from build123d import *

# Parameters (mm, degrees)
CYLINDER001_R     = 1.65
CYLINDER001_DEPTH = 10
CYLINDER002_R     = 1.65
CYLINDER002_DEPTH = 10
CYLINDER003_R     = 1.65
CYLINDER003_DEPTH = 10
CYLINDER004_R     = 1.65
CYLINDER004_DEPTH = 10
CYLINDER_R        = 1.65
CYLINDER_DEPTH    = 10
BOX_W             = 50
BOX_H             = 10
BOX_DEPTH         = 3


with BuildPart() as taladro002:
    # Cylinder001 → Cylinder001 (new body)
    with BuildSketch(Plane(origin=(15, 5, -4), x_dir=(1, 0, 0), z_dir=(0, 0, 1))):
        Circle(CYLINDER001_R)
    extrude(amount=CYLINDER001_DEPTH)


with BuildPart() as taladro003:
    # Cylinder002 → Cylinder002 (new body)
    with BuildSketch(Plane(origin=(25, 5, -4), x_dir=(1, 0, 0), z_dir=(0, 0, 1))):
        Circle(CYLINDER002_R)
    extrude(amount=CYLINDER002_DEPTH)


with BuildPart() as taladro004:
    # Cylinder003 → Cylinder003 (new body)
    with BuildSketch(Plane(origin=(35, 5, -4), x_dir=(1, 0, 0), z_dir=(0, 0, 1))):
        Circle(CYLINDER003_R)
    extrude(amount=CYLINDER003_DEPTH)


with BuildPart() as taladro005:
    # Cylinder004 → Cylinder004 (new body)
    with BuildSketch(Plane(origin=(45, 5, -4), x_dir=(1, 0, 0), z_dir=(0, 0, 1))):
        Circle(CYLINDER004_R)
    extrude(amount=CYLINDER004_DEPTH)


with BuildPart() as taladros:
    # Cylinder → Cylinder (new body)
    with BuildSketch(Plane(origin=(5, 5, -4), x_dir=(1, 0, 0), z_dir=(0, 0, 1))):
        Circle(CYLINDER_R)
    extrude(amount=CYLINDER_DEPTH)

    # Fusion: union taladro002, taladro003, taladro004, taladro005
    add(taladro002.part)
    add(taladro003.part)
    add(taladro004.part)
    add(taladro005.part)


with BuildPart() as pieza_final:
    # Box → Box (new body)
    with BuildSketch(Plane.XY):
        with Locations((25, 5)):
            Rectangle(BOX_W, BOX_H)
    extrude(amount=BOX_DEPTH)

    # Cut: cut Taladros
    add(taladros.part, mode=Mode.SUBTRACT)


solid = pieza_final.part
Read the model definition and answer for the solid it produces. Units are mm, in the model's axes. Give positions to 0.01 mm unless a question says otherwise; leave off trailing zeros. Loops run counter-clockwise (first coordinate to the right, second up) from the corner with the lowest first, then second, coordinate; pieces in that order, holes last. Notation, with made-up numbers: M 87.5,-28.75 L 130.5,-28.75 A19 ccw 130.5,6.25 Z; hole C 41.25,-7.5 d11. An arc over 180 degrees is marked long. Write each question's results on one line, items separated by ' | '.
1. Section C-C on x = 35 is taken. Give the vertices of the cut face in (y, z).
Values:
outline: M 0,0 L 3.35,0 L 3.35,3 L 0,3 Z; M 6.65,0 L 10,0 L 10,3 L 6.65,3 Z
2. Straight lines are drawn through the part: line 1 (X direction, y = 5, z = 2.3); line 2 (Y direction, x = 35, z = 1.95); line 3 (X direction, y = 4.25, z = 2.2). For each, find the intervals that lie inside material, in ascending order. Write a range as [from, to].
Values:
line 1: x = [0, 3.35], [6.65, 13.35], [16.65, 23.35], [26.65, 33.35], [36.65, 43.35], [46.65, 50] | line 2: y = [0, 3.35], [6.65, 10] | line 3: x = [0, 3.53], [6.47, 13.53], [16.47, 23.53], [26.47, 33.53], [36.47, 43.53], [46.47, 50]
3. Section A-A on z = 2.4 is taken. Give the vertices of the cut face in (x, y), plus the area to 3 significant figures.
Values:
outline: M 0,0 L 50,0 L 50,10 L 0,10 Z; hole C 5,5 d3.3; hole C 15,5 d3.3; hole C 25,5 d3.3; hole C 35,5 d3.3; hole C 45,5 d3.3 | area: 457 mm^2
4. Given pin 1 (2 mm diameter, centred on x = 5, y = 5, fed in from -Z) (1 decimal), flat-ended and moving along its own axis, determine where the tip first touches the part or whether it passes through.
Values:
pin 1: passes through
5. The mould has two halves that part along Y. Classify faces 1 (the face through (16.524, 4.368, 1.479)), 2 (the face through (25, 0, 1)), 3 (the face through (50, 5, 1)): pulls with the +Y half, pulls with the -Y half, needs draft (parallel to the pull), parting line crosses it, or undercut.
Values:
face 1: undercut | face 2: pulls with the -Y half | face 3: needs draft
6. Section B-B on y = 5 is taken. Give the vertices of the cut face in (x, z).
Values:
outline: M 0,0 L 3.35,0 L 3.35,3 L 0,3 Z; M 6.65,0 L 13.35,0 L 13.35,3 L 6.65,3 Z; M 16.65,0 L 23.35,0 L 23.35,3 L 16.65,3 Z; M 26.65,0 L 33.35,0 L 33.35,3 L 26.65,3 Z; M 36.65,0 L 43.35,0 L 43.35,3 L 36.65,3 Z; M 46.65,0 L 50,0 L 50,3 L 46.65,3 Z
